Could you check a few things on this model? Use its own coordinates, in mm. A direction names the side the tool comes from. Round coordinates to 2 decimals unless told otherwise and drop trailing zeros. Loops run counter-clockwise (first coordinate to the right, second up) from the corner with the lowest first, then second, coordinate; pieces in that order, holes last. Notation, with made-up numbers: M 64.5,85.5 L 92.5,85.5 A21 cw 92.5,94.5 Z; hole C 60.5,38 d8. An arc over 180 degrees is marked long. One line per item, written item: value. Start each with the question number.
Q1. Thinking about a two-plate mould opening in Z: for faces 4 (the face through (63, -25.4, 65)), 5 (the face through (13, -13, 152.4)), 6 (the face through (22.584, -1.878, 123.783)), which applies, released by +Z, released by -Z, zero draft, split by the parting line, or undercut?
Q2. Please list where these lines run through material, in increasing order: line 1 along X through (y, z) = (-3.5, 90); line 2 along Z through (x, y) = (7, -7); line 3 along Y through (x, z) = (47.5, 54).
Q3. I'm going to push flat-ended pins straight in: pin 1 Ø7.5 at (y, z) = (-13.5, 43) entering from +X; pin 2 Ø10 at (x, z) = (48, 77) entering from -Y; pin 3 Ø1.5 at (y, z) = (-22.5, 83.5) entering from +X. Where does each tip first touch, or does it pass through?
Q4. Imagine slicing it at D-D (z = 52). Please give me the cut outline in (x, y), then the cut area to 3 significant figures.
Q5. Imagine slicing it at A-A (y = -17). Please give me the cut outline in (x, z).
Q6. Imagine slicing it at B-B (z = 101). Please give me the cut outline in (x, y).
Q7. Which directions (+Z, -Z, +X, -X, +Y, -Y) give clear straight access to the entire face, cutting with the end or side of a thin tool? Please do faces 1 (the face through (52.06, -1.88, 70.47)), 2 (the face through (13, -13, 148.59)), 3 (the face through (35, 0, 71)).
Q8. Imagine slicing it at C-C (x = 69.5). Please give me the cut outline in (y, z).
from build123d import *

# Parameters (mm, degrees)
F1_DEPTH = 25.4
F3_DEPTH = 3.81
F4_R     = 5.08
F5_R     = 1.27


with BuildPart() as f1:
    # F0 (on Front) → F1 (new body)
    with BuildSketch(Plane.XZ):
        Polygon((0, 152.4), (0, 0), (97.536, 0), (25.4, 152.4), align=None)
        Polygon((3.81, 3.81), (3.81, 148.59), (22.9881477466, 148.59), (91.5173477466, 3.81), align=None, mode=Mode.SUBTRACT)
    extrude(amount=F1_DEPTH)

    # F2 (on face) → F3 (join)
    with BuildSketch(Plane(origin=(0, 0, 0), x_dir=(-1, 0, 0), z_dir=(0, 1, 0))):
        Polygon((-39.4677877212, 66.6927195413), (-56.4292804153, 77.939719714), (-58.0762150779, 74.460280286), (-40.9881443162, 63.1293474326), (-88.6470719162, 9.873963022), (-91.5173477466, 3.81), (-88.9609051741, 3.81), (-41.0075535603, 57.3943818268), (-49.5929707574, 3.81), (-45.7343769892, 3.81), (-37.0705642602, 57.8836738464), (-6.0069643909, 3.81), (-3.81, 3.81), (-3.81, 7.6343454213), (-35.3261969761, 62.4958734908), (-3.81, 74.1685390375), (-3.81, 78.2314609625), (-34.7235350429, 66.7820035392), (-3.81, 143.4933682752), (-3.81, 148.59), (-5.863866516, 148.59), (-25.7159540879, 99.3274123216), (-11.4154306532, 148.59), (-15.3827170934, 148.59), (-29.9899241521, 98.2709454732), (-21.0533379782, 148.59), (-22.9881477466, 148.59), (-26.0848739491, 142.0476206988), align=None)
    extrude(amount=-F3_DEPTH)

    # F4
    f4_edges = [f1.edges().sort_by_distance(p)[0] for p in [
        (40.988144, -1.905, 63.129347),
        (41.007554, -1.905, 57.394382),
        (35.326197, -1.905, 62.495873),
        (37.070564, -1.905, 57.883674),
        (39.467788, -1.905, 66.69272),
        (34.723535, -1.905, 66.782004),
    ]]
    fillet(f4_edges, radius=F4_R)

    # F5
    f5_edges = [f1.edges().sort_by_distance(p)[0] for p in [
        (25.715954, -1.905, 99.327412),
    ]]
    fillet(f5_edges, radius=F5_R)


solid = f1.part
Report:
1. face 4: zero draft
1. face 5: released by +Z
1. face 6: undercut
2. line 1: x = 0 to 3.81, 25.37 to 35.33, 50.72 to 54.94
2. line 2: z = 0 to 3.81, 148.59 to 152.4
2. line 3: y = -3.81 to 0
3. pin 1: stops at x = 78.96
3. pin 2: stops at y = -3.81
3. pin 3: stops at x = 58.37
4. outline: M 0,-25.4 L 3.81,-25.4 L 3.81,0 L 0,0 Z; M 29.3,-3.81 L 50.95,-3.81 L 50.95,0 L 29.3,0 Z; M 68.71,-25.4 L 72.92,-25.4 L 72.92,0 L 68.71,0 Z
4. area: 286 mm²
5. outline: M 0,0 L 97.54,0 L 25.4,152.4 L 0,152.4 Z; hole M 3.81,3.81 L 91.52,3.81 L 22.99,148.59 L 3.81,148.59 Z
6. outline: M 0,-25.4 L 3.81,-25.4 L 3.81,0 L 0,0 Z; M 20.93,-3.81 L 29.2,-3.81 L 29.2,0 L 20.93,0 Z; M 29.51,-3.81 L 33.37,-3.81 L 33.37,0 L 29.51,0 Z; M 45.51,-25.4 L 49.73,-25.4 L 49.73,0 L 45.51,0 Z
7. face 1: +Y, -Y
7. face 2: -Y
7. face 3: +Z, -Z, +X, -X, +Y
8. outline: M -25.4,0 L 0,0 L 0,3.81 L -25.4,3.81 Z; M -25.4,50.33 L 0,50.33 L 0,59.23 L -25.4,59.23 Z; M -3.81,25.56 L 0,25.56 L 0,31.27 L -3.81,31.27 Z
